Here's how the part is built. I have some questions about the finished solid (model axes, mm). Face numbers are marked on the shaded views. A direction names the side the tool comes from. Coordinates: 2 decimals unless noted, no trailing zeros. Write each loop counter-clockwise with the first axis right and the second up, starting at its lowest first coordinate (ties: lowest second). Pieces come first, ordered by that corner, then holes. Notation, with made-up numbers: (15, -24) -> (21, -24) arc R38 ccw to (21, 14) -> close; hole circle Ø9 at (25.25, 41). An arc over 180 degrees is marked (long way). Answer in a Markdown table with one row per item. Add a question column.
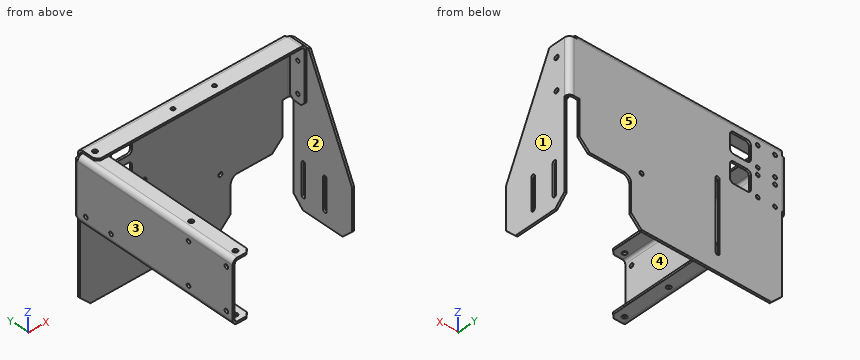
from build123d import *

# Parameters (mm, degrees)
ODGI_CIE_BAZOWE1_DEPTH                            = 37.5
ODGI_CIE_KRAW_DZI1_DEPTH                          = 296
ODGI_CIE_KRAW_DZI2_DEPTH                          = 246
ODGI_CIE_KRAW_DZI2_BEND_DEPTH                     = 246
OTW_R_POD_RUB_M51_D                               = 5.8
OTW_R_POD_RUB_M51_DEPTH                           = 10
OTW_R_POD_RUB_M51_TIP                             = 1.742495795
OTW_R_POD_RUB_M61_D                               = 6.6
ODGI_CIE_KRAW_DZI3_DEPTH                          = 79
SZKIC38_W                                         = 293
SZKIC38_H                                         = 130
WYPUST1_DEPTH                                     = 3
WYPUST2_DEPTH                                     = 3
ODGI_CIE_KRAW_DZI4_DEPTH                          = 23
SZKIC49_R                                         = 3
WYTNIJ_WYCI_GNI_CIE1_DEPTH                        = 351.991809021
SZCZELINA_START                                   = 159
SZCZELINA_POD_RUB_M53_DEPTH                       = 3
SFAZOWANIE3_SIZE                                  = 5
POG_BIENIE_WALCOWE_POD_M5_RUB_Z_BEM_S_D           = 5.5
POG_BIENIE_WALCOWE_POD_M5_RUB_Z_BEM_S_DEPTH       = 10
POG_BIENIE_WALCOWE_POD_M5_RUB_Z_BEM_S_CBORE_D     = 6.5
POG_BIENIE_WALCOWE_POD_M5_RUB_Z_BEM_S_CBORE_DEPTH = 3.7
POG_BIENIE_WALCOWE_POD_M5_RUB_Z_BEM_S_TIP         = 1.652366702
POG_BIENIE_WALCOWE_POD_M5_RUB_Z_B_2_D             = 5.5
POG_BIENIE_WALCOWE_POD_M5_RUB_Z_B_2_DEPTH         = 10
POG_BIENIE_WALCOWE_POD_M5_RUB_Z_B_2_CBORE_D       = 6.5
POG_BIENIE_WALCOWE_POD_M5_RUB_Z_B_2_CBORE_DEPTH   = 3.7
POG_BIENIE_WALCOWE_POD_M5_RUB_Z_B_2_TIP           = 1.652366702
SZKIC57_W                                         = 75
SZKIC57_H                                         = 65
WYTNIJ_WYCI_GNI_CIE2_DEPTH                        = 10
WYTNIJ_WYCI_GNI_CIE3_REACH                        = 352.992
SZKIC58_W                                         = 30
SZKIC58_H                                         = 30
SZYK_LINIOWY1_COUNT                               = 2
SZYK_LINIOWY1_PITCH                               = 40
SFAZOWANIE4_SIZE                                  = 15
ZAOKR_GLENIE1_R                                   = 10
ZAOKR_GLENIE2_R                                   = 5
OTW_R_POD_RUB_M52_D                               = 5.5
OTW_R_POD_RUB_M52_DEPTH                           = 10
OTW_R_POD_RUB_M52_TIP                             = 1.652366702
OTW_R_POD_RUB_M53_D                               = 5.5
OTW_R_POD_RUB_M53_DEPTH                           = 10
OTW_R_POD_RUB_M53_TIP                             = 1.652366702


# Read off the part's stored shape, not the designer's step: Szczelina pod śrubę M53
# Sheet-metal steps are written as plain solids
with BuildPart() as part:
    # Szkic1 → Odgięcie bazowe1 (new, symmetric)
    with BuildSketch(Plane.XY):
        with BuildLine():
            Line((-150, -250), (-150, -4))
            ThreePointArc((-150, -4), (-148.828427125, -1.171572875), (-146, 0))
            Line((-146, 0), (150, 0))
            Line((150, 0), (150, 3))
            Line((150, 3), (-146, 3))
            ThreePointArc((-146, 3), (-150.949747468, 0.949747468), (-153, -4))
            Line((-153, -4), (-153, -250))
            Line((-153, -250), (-150, -250))
        make_face()
    extrude(amount=ODGI_CIE_BAZOWE1_DEPTH, both=True)

    # Odgięcie krawędzi1 section (across the edge) → Odgięcie krawędzi1 (add)
    with BuildSketch(Plane(origin=(150, 0, 45.5), x_dir=(0, 0, -1), z_dir=(-1, 0, 0))):
        with BuildLine():
            Line((-3, 4), (-3, 27))
            Line((-3, 27), (0, 27))
            Line((0, 27), (0, 4))
            ThreePointArc((0, 4), (1.171572875, 1.171572875), (4, 0))
            Line((4, 0), (8, 0))
            Line((8, 0), (8, -3))
            Line((8, -3), (4, -3))
            ThreePointArc((4, -3), (-0.949747468, -0.949747468), (-3, 4))
        make_face()
    extrude(amount=ODGI_CIE_KRAW_DZI1_DEPTH)

    # Odgięcie krawędzi2 section (across the edge) → Odgięcie krawędzi2 (add)
    with BuildSketch(Plane(origin=(-150, -4, 41.5), x_dir=(0, 0, -1), z_dir=(0, -1, 0))):
        with BuildLine():
            Line((-3, 4), (-3, 22))
            Line((-3, 22), (0, 22))
            Line((0, 22), (0, 4))
            ThreePointArc((0, 4), (1.171572875, 1.171572875), (4, 0))
            Line((4, 0), (4, -3))
            ThreePointArc((4, -3), (-0.949747468, -0.949747468), (-3, 4))
        make_face()
    extrude(amount=ODGI_CIE_KRAW_DZI2_DEPTH)

    # Odgięcie krawędzi2 section 2 (across the edge) → Odgięcie krawędzi2 bend (add)
    with BuildSketch(Plane(origin=(-150, -250, -41.5), x_dir=(0, 0, 1), z_dir=(0, 1, 0))):
        with BuildLine():
            Line((-3, 4), (-3, 22))
            Line((-3, 22), (0, 22))
            Line((0, 22), (0, 4))
            ThreePointArc((0, 4), (1.171572875, 1.171572875), (4, 0))
            Line((4, 0), (4, -3))
            ThreePointArc((4, -3), (-0.949747468, -0.949747468), (-3, 4))
        make_face()
    extrude(amount=ODGI_CIE_KRAW_DZI2_BEND_DEPTH)

    # Otwór pod śrubę M51
    with Locations(Plane.ZY.offset(153)):
        with Locations((-30, -240), (30, -240), (-30, -180), (30, -180), (-30, -17), (-30, -57)):
            Hole(OTW_R_POD_RUB_M51_D / 2, depth=OTW_R_POD_RUB_M51_DEPTH)
            with Locations((0, 0, -(OTW_R_POD_RUB_M51_DEPTH + OTW_R_POD_RUB_M51_TIP / 2))):  # 118° drill point
                Cone(0, OTW_R_POD_RUB_M51_D / 2, OTW_R_POD_RUB_M51_TIP, mode=Mode.SUBTRACT)

    # Otwór pod śrubę M61 (through all)
    with Locations(Plane.XY.offset(44.5)):
        with Locations((-140, -240), (-140, -170)):
            Hole(OTW_R_POD_RUB_M61_D / 2)

    # Odgięcie krawędzi3 section (across the edge) → Odgięcie krawędzi3 (add)
    with BuildSketch(Plane(origin=(159, 0, -37.5), x_dir=(-1, 0, 0), z_dir=(0, 0, 1))):
        with BuildLine():
            Line((-3, 4), (-3, 28))
            Line((-3, 28), (0, 28))
            Line((0, 28), (0, 4))
            ThreePointArc((0, 4), (1.171572875, 1.171572875), (4, 0))
            Line((4, 0), (9, 0))
            Line((9, 0), (9, -3))
            Line((9, -3), (4, -3))
            ThreePointArc((4, -3), (-0.949747468, -0.949747468), (-3, 4))
        make_face()
    extrude(amount=ODGI_CIE_KRAW_DZI3_DEPTH)

    # Szkic38 → Wypust1 (add)
    with BuildSketch(Plane(origin=(0, 3, 0), x_dir=(1, 0, 0), z_dir=(0, 1, 0))):
        with Locations((0.5, 102.5)):
            Rectangle(SZKIC38_W, SZKIC38_H)
    extrude(amount=-WYPUST1_DEPTH)

    # Szkic41 → Wypust2 (add)
    with BuildSketch(Plane(origin=(162, 0, 0), x_dir=(0, 0, -1), z_dir=(1, 0, 0))):
        Polygon((37.5, -4), (181.5, -4), (181.5, -97.00689818), (106.5, -97.00689818), (-41.5, -28), (37.5, -28), align=None)
    extrude(amount=-WYPUST2_DEPTH)

    # Odgięcie krawędzi4 section (across the edge) → Odgięcie krawędzi4 (add)
    with BuildSketch(Plane(origin=(154, -4, 45.5), x_dir=(-1, 0, 0), z_dir=(0, -1, 0))):
        with BuildLine():
            Line((-3, 4), (-3, 81))
            Line((-3, 81), (0, 81))
            Line((0, 81), (0, 4))
            ThreePointArc((0, 4), (1.171572875, 1.171572875), (4, 0))
            Line((4, 0), (4, -3))
            ThreePointArc((4, -3), (-0.949747468, -0.949747468), (-3, 4))
        make_face()
    extrude(amount=ODGI_CIE_KRAW_DZI4_DEPTH)

    # Szkic49 → Wytnij-wyciągnięcie1 (cut, through all)
    with BuildSketch(Plane(origin=(0, 3, 0), x_dir=(1, 0, 0), z_dir=(0, 1, 0))):
        with Locations(Location((57, 91.5, 0), (0, 0, 270))):
            Circle(SZKIC49_R)
        with BuildLine():
            Line((-50, 141.5), (-50, 41.5))
            ThreePointArc((-50, 41.5), (-53, 38.5), (-56, 41.5))
            Line((-56, 41.5), (-56, 141.5))
            ThreePointArc((-56, 141.5), (-53, 144.5), (-50, 141.5))
        make_face()
    extrude(amount=-WYTNIJ_WYCI_GNI_CIE1_DEPTH, mode=Mode.SUBTRACT)

    # Szczelina pod śrubę M53 outline → Szczelina pod śrubę M53 (cut)
    with BuildSketch(Plane.YZ.offset(SZCZELINA_START)):
        with BuildLine():
            Line((-56.75, -117.75), (-56.75, -162.25))
            ThreePointArc((-56.75, -162.25), (-54, -165), (-51.25, -162.25))
            Line((-51.25, -162.25), (-51.25, -117.75))
            ThreePointArc((-51.25, -117.75), (-54, -115), (-56.75, -117.75))
        make_face()
        with BuildLine():
            ThreePointArc((-22.75, -162.25), (-20, -165), (-17.25, -162.25))
            Line((-17.25, -162.25), (-17.25, -117.75))
            ThreePointArc((-17.25, -117.75), (-20, -115), (-22.75, -117.75))
            Line((-22.75, -117.75), (-22.75, -162.25))
        make_face()
    extrude(amount=SZCZELINA_POD_RUB_M53_DEPTH, mode=Mode.SUBTRACT)

    # Sfazowanie3
    sfazowanie3_edges = [part.edges().sort_by_distance(p)[0] for p in [
        (155.5, -4, -35.5),
        (155.5, -27, -35.5),
        (-146, -27, 47),
        (-128, -4, 43),
        (-128, -250, 43),
        (-128, -250, -43),
        (-128, -4, -43),
    ]]
    chamfer(sfazowanie3_edges, length=SFAZOWANIE3_SIZE)

    # Pog_bienie walcowe pod M5 _rub_ z _bem s
    with Locations(Plane.XY.offset(48.5)):
        with Locations((-137, -14)):
            CounterBoreHole(POG_BIENIE_WALCOWE_POD_M5_RUB_Z_BEM_S_D / 2, POG_BIENIE_WALCOWE_POD_M5_RUB_Z_BEM_S_CBORE_D / 2, POG_BIENIE_WALCOWE_POD_M5_RUB_Z_BEM_S_CBORE_DEPTH, depth=POG_BIENIE_WALCOWE_POD_M5_RUB_Z_BEM_S_DEPTH)
            with Locations((0, 0, -(POG_BIENIE_WALCOWE_POD_M5_RUB_Z_BEM_S_DEPTH + POG_BIENIE_WALCOWE_POD_M5_RUB_Z_BEM_S_TIP / 2))):  # 118° drill point
                Cone(0, POG_BIENIE_WALCOWE_POD_M5_RUB_Z_BEM_S_D / 2, POG_BIENIE_WALCOWE_POD_M5_RUB_Z_BEM_S_TIP, mode=Mode.SUBTRACT)

    # Pog_bienie walcowe pod M5 _rub_ z _b 2
    with Locations(Plane(origin=(162, 0, 0), x_dir=(0, 0, -1), z_dir=(1, 0, 0))):
        with Locations((-21.5, -16.600519764), (23.5, -16.600519764)):
            CounterBoreHole(POG_BIENIE_WALCOWE_POD_M5_RUB_Z_B_2_D / 2, POG_BIENIE_WALCOWE_POD_M5_RUB_Z_B_2_CBORE_D / 2, POG_BIENIE_WALCOWE_POD_M5_RUB_Z_B_2_CBORE_DEPTH, depth=POG_BIENIE_WALCOWE_POD_M5_RUB_Z_B_2_DEPTH)
            with Locations((0, 0, -(POG_BIENIE_WALCOWE_POD_M5_RUB_Z_B_2_DEPTH + POG_BIENIE_WALCOWE_POD_M5_RUB_Z_B_2_TIP / 2))):  # 118° drill point
                Cone(0, POG_BIENIE_WALCOWE_POD_M5_RUB_Z_B_2_D / 2, POG_BIENIE_WALCOWE_POD_M5_RUB_Z_B_2_TIP, mode=Mode.SUBTRACT)

    # Szkic57 → Wytnij-wyciągnięcie2 (cut)
    with BuildSketch(Plane(origin=(0, 3, 0), x_dir=(1, 0, 0), z_dir=(0, 1, 0))):
        with Locations((109.5, 135)):
            Rectangle(SZKIC57_W, SZKIC57_H)
    extrude(amount=-WYTNIJ_WYCI_GNI_CIE2_DEPTH, mode=Mode.SUBTRACT)

    # Szkic58 → Wytnij-wyciągnięcie3 (cut, up to next)
    with BuildSketch(Plane(origin=(0, 3, 0), x_dir=(1, 0, 0), z_dir=(0, 1, 0)), mode=Mode.PRIVATE) as wytnij_wyci_gni_cie3_sk1:
        with Locations((-86, -18.5)):
            Rectangle(SZKIC58_W, SZKIC58_H)
    wytnij_wyci_gni_cie3_tool1 = extrude(wytnij_wyci_gni_cie3_sk1.sketch, amount=-WYTNIJ_WYCI_GNI_CIE3_REACH, mode=Mode.PRIVATE) & part.part
    wytnij_wyci_gni_cie3 = wytnij_wyci_gni_cie3_tool1.solids().sort_by_distance((-86, 3, 18.5))[0]
    add(wytnij_wyci_gni_cie3, mode=Mode.SUBTRACT)

    # Szyk liniowy1: Wytnij-wyciągnięcie3 ×2
    with Locations(*[(0, 0, -i * SZYK_LINIOWY1_PITCH) for i in range(1, SZYK_LINIOWY1_COUNT)]):
        add(wytnij_wyci_gni_cie3, mode=Mode.SUBTRACT)

    # Sfazowanie4
    sfazowanie4_edges = [part.edges().sort_by_distance(p)[0] for p in [
        (-146, 1.5, -167.5),
        (160.5, -4, -181.5),
        (160.5, -97.00689818, -181.5),
        (147, 1.5, -102.5),
        (72, 1.5, -167.5),
    ]]
    chamfer(sfazowanie4_edges, length=SFAZOWANIE4_SIZE)

    # Zaokrąglenie1
    zaokr_glenie1_edges = [part.edges().sort_by_distance(p)[0] for p in [
        (72, 1.5, -102.5),
    ]]
    fillet(zaokr_glenie1_edges, radius=ZAOKR_GLENIE1_R)

    # Zaokrąglenie2
    zaokr_glenie2_edges = [part.edges().sort_by_distance(p)[0] for p in [
        (-101, 1.5, 33.5),
        (-101, 1.5, 3.5),
        (-71, 1.5, 3.5),
        (-71, 1.5, 33.5),
        (-101, 1.5, -6.5),
        (-101, 1.5, -36.5),
        (-71, 1.5, -36.5),
        (-71, 1.5, -6.5),
    ]]
    fillet(zaokr_glenie2_edges, radius=ZAOKR_GLENIE2_R)

    # Otwór pod śrubę M52
    with Locations(Plane(origin=(0, 3, 0), x_dir=(1, 0, 0), z_dir=(0, 1, 0))):
        with Locations((-111, 36.5), (-111, -3.5), (-111, 6.5), (-111, -33.5), (-136, 36.5), (-136, -3.5), (-136, 6.5), (-136, -33.5)):
            Hole(OTW_R_POD_RUB_M52_D / 2, depth=OTW_R_POD_RUB_M52_DEPTH)
            with Locations((0, 0, -(OTW_R_POD_RUB_M52_DEPTH + OTW_R_POD_RUB_M52_TIP / 2))):  # 118° drill point
                Cone(0, OTW_R_POD_RUB_M52_D / 2, OTW_R_POD_RUB_M52_TIP, mode=Mode.SUBTRACT)

    # Otwór pod śrubę M53
    with Locations(Plane.XY.offset(48.5)):
        with Locations((-25.078617212, -15), (34.921382788, -15)):
            Hole(OTW_R_POD_RUB_M53_D / 2, depth=OTW_R_POD_RUB_M53_DEPTH)
            with Locations((0, 0, -(OTW_R_POD_RUB_M53_DEPTH + OTW_R_POD_RUB_M53_TIP / 2))):  # 118° drill point
                Cone(0, OTW_R_POD_RUB_M53_D / 2, OTW_R_POD_RUB_M53_TIP, mode=Mode.SUBTRACT)


solid = part.part
Q1. Imagine slicing it at A-A on x = 136.5. Please give me the cut outline in (y, z), plus the area to 3 significant figures.
Q2. If we mould it in two halves opening along X, with no side actions, what happens to the marked faces 1, 2 and 3? For each: pulls with the +X half, pulls with the -X half, needs draft (parallel to the pull), parting line crosses it, or undercut.
Q3. I'm going to push flat-ended pins straight in: P1, Ø0.9, axis at y = 1, z = -97, coming from the -X side; P2, Ø9, axis at x = -139.5, y = -140, coming from the -Z side; P3, Ø18.5, axis at x = -20, y = -16.5, coming from the -Z side. Where does each tip first touch, or does it pass through?
Q4. I need wall thicknesses on line 1 (Y direction, x = -140, z = 42); line 2 (Z direction, x = -66, y = -13); line 3 (Y direction, x = -101, z = -164). Which ranges of each line are inside material? Lowest first, please. Write a range as [from, to].
Q5. Imagine slicing it at B-B on y = -232.5. Please give me the cut outline in (x, z), plus the area to 3 significant figures.
Q6. For the marked faces 4 and 5, which set-ups out of +Z, -Z, +X, -X, +Y, -Y let a thin tool reach every point of the face, with its end or its side?
Q7. Imagine slicing it at C-C on x = -61. Please give me the cut outline in (y, z), plus the area to 3 significant figures.
Result sheet:
| question | item | result |
|---|---|---|
| 1 | outline | (-27, 45.5) -> (-4, 45.5) arc R4 cw to (0, 41.5) -> (0, -98) -> (3, -98) -> (3, 41.5) arc R7 ccw to (-4, 48.5) -> (-27, 48.5) -> close |
| 1 | area | 513 mm^2 |
| 2 | face 1 | pulls with the +X half |
| 2 | face 2 | undercut |
| 2 | face 3 | pulls with the -X half |
| 3 | P1 | stops at x = -146 |
| 3 | P2 | stops at z = -44.5 |
| 3 | P3 | stops at z = 45.5 |
| 4 | line 1 | y = [-250, -243.3], [-236.7, -173.3], [-166.7, -4], [-0.03, 2.98] |
| 4 | line 2 | z = [45.5, 48.5] |
| 4 | line 3 | y = [0, 3] |
| 5 | outline | (-153, -37.5) arc R7 ccw to (-146, -44.5) -> (-128, -44.5) -> (-128, -41.5) -> (-146, -41.5) arc R4 cw to (-150, -37.5) -> (-150, 37.5) arc R4 cw to (-146, 41.5) -> (-128, 41.5) -> (-128, 44.5) -> (-146, 44.5) arc R7 ccw to (-153, 37.5) -> close |
| 5 | area | 385 mm^2 |
| 6 | face 4 | -Y |
| 6 | face 5 | +Z, -Z, +X, -X, +Y |
| 7 | outline | (-27, 45.5) -> (-4, 45.5) arc R4 cw to (0, 41.5) -> (0, -167.5) -> (3, -167.5) -> (3, 41.5) arc R7 ccw to (-4, 48.5) -> (-27, 48.5) -> close |
| 7 | area | 722 mm^2 |
